Check sheet for the drawn part. Datum: minimum x, y, z corner. Units: mm. A direction names the side the tool comes from. Coordinates: 2 decimals unless noted, no trailing zeros. Order: outer loops, then holes, each group sorted by start corner. A loop starts at its lowest first (then second) coordinate and runs counter-clockwise, first axis right, second up. Notation, with made-up numbers: M -16.5,35.25 L 12.5,35.25 A14 ccw 12.5,48.25 Z; hole C 32,-9.5 d8. An arc over 180 degrees is marked long. Return JSON: item names as keys, results as strings. Group by question number.
Q1. Thickness scan on probe 1 along Z at (x, y) = (49.5, 92.5) (1 decimal); probe 2 along Z at (x, y) = (123, 101); probe 3 along X at (y, z) = (92, 154) (1 decimal). Record the ranges inside material, lowest first.
Q2. Section check A-A, the plane y = 90. Enter the section's corners in (x, z) (1 decimal).
Q3. Section check D-D, the plane y = 36. Enter the section's corners in (x, z).
Q4. Go/stop test with flat-tipped pins: pin 1 Ø10 at (x, y) = (76.5, 47) entering from +Z; pin 2 Ø6 at (x, z) = (171.5, 218) entering from -Y; pin 3 Ø3 at (x, y) = (71, 68.5) entering from -Z. Record where each tip stops, or that it passes through.
Q5. Mould release check, pull along X, two halves, no side actions. Record for the marked faces 1, 2 and 3: pulls with the +X half, pulls with the -X half, needs draft (parallel to the pull), parting line crosses it, or undercut.
Q6. Section check B-B, the plane x = 127. Enter the section's corners in (y, z), then the cut area to 3 significant figures.
Q7. Access from +Z, -Z, +X, -X, +Y, -Y to the whole of each face (thin tool, end or side, straight path). Record for the marked faces 4, 5, 6 and 7.
Q8. Section check C-C, the plane z = 137. Enter the section's corners in (x, y) (1 decimal).
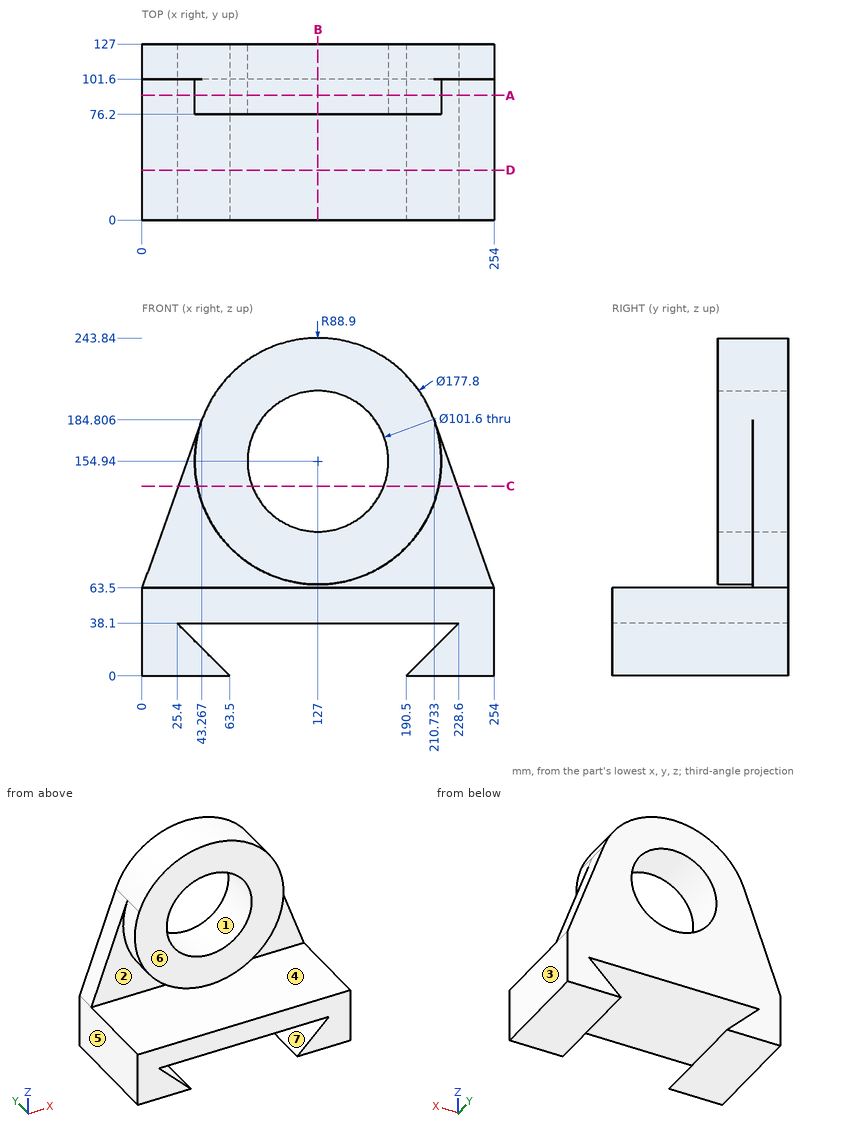
Numbers:
{
 "1": {"probe 1": "z = 0 to 14, 38.1 to 63.5, 111.4 to 198.5", "probe 2": "z = 38.1 to 63.5, 66.13 to 104.3, 205.58 to 243.75", "probe 3": "x = 38.1 to 76.2, 177.8 to 215.9"},
 "2": {"outline": "M 0,0 L 63.5,0 L 25.4,38.1 L 228.6,38.1 L 190.5,0 L 254,0 L 254,63.5 L 0,63.5 Z; M 210.7,184.8 A88.9 ccw long 215.9,154.9 A88.9 ccw Z; hole C 127,154.9 d101.6"},
 "3": {"outline": "M 0,0 L 63.5,0 L 25.4,38.1 L 228.6,38.1 L 190.5,0 L 254,0 L 254,63.5 L 0,63.5 Z"},
 "4": {"pin 1": "stops at z = 63.5", "pin 2": "stops at y = 76.2", "pin 3": "stops at z = 38.1"},
 "5": {"face 1": "undercut", "face 2": "needs draft", "face 3": "pulls with the +X half"},
 "6": {"outline": "M 0,38.1 L 127,38.1 L 127,104.14 L 76.2,104.14 L 76.2,66.04 L 101.6,66.04 L 101.6,63.5 L 0,63.5 Z; M 76.2,205.74 L 127,205.74 L 127,243.84 L 76.2,243.84 Z", "area": "7,160 mm2"},
 "7": {"face 4": "+X, -X, -Y", "face 5": "+Z, -Z, -X, +Y, -Y", "face 6": "+Z, +X, -X, -Y", "face 7": "+Y, -Y"},
 "8": {"outline": "M 26.2,101.6 L 39.9,101.6 L 39.9,76.2 L 79.5,76.2 L 79.5,127 L 26.2,127 Z; M 174.5,76.2 L 214.1,76.2 L 214.1,101.6 L 227.8,101.6 L 227.8,127 L 174.5,127 Z"}
}
